Can you work these out from the model? Positions are in its coordinate system, mm. Give positions to 0.01 mm unless a question says otherwise; leave off trailing zeros. Write each loop counter-clockwise with the first axis right and the second up, starting at its lowest first coordinate (ties: lowest second). Pieces come first, ordered by that corner, then holes.
Autodesk Inventor part; units mm, degrees
ref_plane "YZ Plane" through (0, 0, 0) normal (1, 0, 0) x (0, 1, 0)
ref_plane "XZ Plane" through (0, 0, 0) normal (0, 1, 0) x (-1, 0, 0)
ref_plane "XY Plane" through (0, 0, 0) normal (0, 0, 1) x (1, 0, 0)
sketch "Sketch1" plane through (0, 0, 0) normal (0, 1, 0) x (-1, 0, 0)
  line L0 (0, 0) -> (-12.7, 0)
  line L1 (0, 0) -> (12.7, 0)
  line L2 (38.1, 25.4) -> (38.1, 355.6)
  line L3 (12.7, 381) -> (0, 381)
  line L4 (38.1, 355.6) -> (12.7, 381)
  line L5 (38.1, 25.4) -> (12.7, 0)
  circle A0 centre (31.75, 184.15) radius 2.2225
  circle A1 centre (-6.35, 19.05) radius 2.2225
  circle A2 centre (-19.05, 19.05) radius 2.2225
  circle A3 centre (-6.35, 361.95) radius 2.2225
  circle A4 centre (-19.05, 361.95) radius 2.2225
  line L6 (-6.35, 0) -> (0, 0)
  line L7 (0, 381) -> (-19.05, 381)
  line L8 (-44.45, 355.6) -> (-44.45, 25.4)
  line L9 (-19.05, 0) -> (0, 0)
  arc A5 (-19.05, 381) -> (-44.45, 355.6) centre (-19.05, 355.6) ccw
  arc A6 (-44.45, 25.4) -> (-19.05, 0) centre (-19.05, 25.4) ccw
  point P0 (38.1, 381)
  point P1 (38.1, 0)
  point P2 (-44.45, 0)
  point P3 (-44.45, 381)
  dimension "d2" = 38.1
  dimension "d3" = 381
  dimension "d5" = 25.4
  dimension "d6" = 25.4
  dimension "d7" = 25.4
  dimension "d8" = 25.4
  dimension "d12" = 4.445
  dimension "d13" = 4.445
  dimension "d14" = 4.445
  dimension "d15" = 4.445
  dimension "d16" = 4.445
  dimension "d20" = 44.45
  dimension "d21" = 381
  dimension "d22" = 25.4
extrude "Extrusion1" add sketch "Sketch1" along normal blind 1.778
properties part number "side_ring_guard_piece"
(1) Imagine slicing it at A-A, the plane y = 0.95. Give the number of separate pieces and of enclosed holes in the cut face, plus the area to 3 significant figures.
Returned:
separate pieces: 1
enclosed holes: 5
area: 30,500 mm2
(2) Imagine slicing it at B-B, the plane x = -20.5. Write out the boundary of the cut face in (y, z), plus the area to 3 significant figures.
Returned:
outline: (0, 7.8) - (1.78, 7.8) - (1.78, 373.2) - (0, 373.2) - close
area: 650 mm2
(3) If I drill on L1, parallel to Z at x = 19.05, y = 1.1; L2, parallel to X at y = 0.95, z = 184.15; L3, parallel to X at y = 1.1, z = 361.95, over which ranges is the centre line in solid material (lowest first)?
Returned:
L1: z = 0 to 16.83, 21.27 to 359.73, 364.17 to 381
L2: x = -38.1 to -33.97, -29.53 to 44.45
L3: x = -31.75 to 4.13, 8.57 to 16.83, 21.27 to 43.64
(4) Will this pin go through, and if not, where does the flat tip stop? P1, Ø6, axis at x = -31.75, z = 184.15, coming from the -Y side.
Returned:
P1: stops at y = 0
